Autodesk Inventor part; units mm, degrees
ref_plane "YZ Plane" through (0, 0, 0) normal (1, 0, 0) x (0, 1, 0)
ref_plane "XZ Plane" through (0, 0, 0) normal (0, 1, 0) x (-1, 0, 0)
ref_plane "XY Plane" through (0, 0, 0) normal (0, 0, 1) x (1, 0, 0)
ref_plane "Plano de trabajo1" through (0, 0, 0) normal (0, 0, -1) x (-1, 0, 0)
sketch "Boceto4" plane through (0, 0, 0) normal (0, 0, -1) x (-1, 0, 0)
  circle A0 centre (0, 0) radius 5
  circle A1 centre (0, 0) radius 10
  dimension "d16" = 20
extrude "Extrusión2" add sketch "Boceto4" along normal blind 40
sketch "Boceto5" plane through (0, 0, -40) normal (0, 0, -1) x (-1, 0, 0)
  arc A0 (-15, 0) -> (15, 0) centre (0, 0) ccw
  line L0 (-72.8349, 131.1538) -> (-42.8349, 79.1923)
  line L1 (-47.1651, 76.6923) -> (-77.1651, 128.6538)
  arc A1 (-72.8349, 131.1538) -> (-77.1651, 128.6538) centre (-75, 129.9038) ccw
  arc A2 (-70.4175, 131.9041) -> (-79.3301, 127.4038) centre (-75, 129.9038) ccw
  arc A3 (-47.1651, 76.6923) -> (-42.8349, 79.1923) centre (-45, 77.9423) ccw
  arc A4 (-15, 0) -> (15, 0) centre (0, 0) ccw
  arc A5 (-13.6856, -6.1404) -> (12.4137, 8.4202) centre (0, 0) ccw
  line L2 (-79.3301, 127.4038) -> (-13.2209, -7.0857)
  line L3 (-70.4175, 131.9041) -> (12.5, 8.2916)
  circle A6 centre (0, 0) radius 5
  point P0 (-13.2209, -7.0857)
  point P1 (15, 0)
  point P2 (12.5, 8.2916)
extrude "Extrusión3" add sketch "Boceto5" along normal blind 3 contours L2 A2 L3 A5 A0
sketch "Boceto10" plane through (0, 0, 0) normal (0, 0, -1) x (-1, 0, 0)
  arc A0 (-10, 0) -> (10, 0) centre (0, 0) ccw
  circle A1 centre (0, 0) radius 10
  line L0 (-10, 0) -> (-10, 10)
  line L1 (-10, 10) -> (10, 10)
  line L2 (10, 10) -> (10, 0)
  circle A2 centre (0, 0) radius 5
  dimension "d29" = 10
extrude "Extrusión5" add sketch "Boceto10" against normal blind 10
sketch "Boceto11" plane through (-10, 10, 0) normal (0, 1, 0) x (1, 0, 0)
  circle A0 centre (10, -5) radius 5
  point P0 (10, 0)
extrude "Extrusión6" add sketch "Boceto11" along normal blind 480
sketch "Boceto12" plane through (0, 490, 5) normal (0, 1, 0) x (1, 0, 0)
  arc A0 (25, 0) -> (-25, 0) centre (0, 0) ccw
  line L0 (25, 0) -> (-25, 0)
  point P0 (0, 5)
revolve "Revolución1" add sketch "Boceto12" angle 360 about axis through (25, 490, 5) along (-1, 0, 0)
properties part number "Palanca"
The listing builds one solid part. Answer for the finished solid, in the listing's coordinates (mm). A direction names the side the tool comes from. Coordinates: 2 decimals unless noted, no trailing zeros. Write each loop counter-clockwise with the first axis right and the second up, starting at its lowest first coordinate (ties: lowest second). Pieces come first, ordered by that corner, then holes. Notation, with made-up numbers: (-37, -31.75) - (-13, -31.75) arc R27 cw to (-13, 3.25) - close; hole circle Ø6 at (54.5, 16.5). An arc over 180 degrees is marked (long way). Put each result on its own line as item: value.
1. The part is cut by section D-D on z = -15.5. Give the vertices of the cut face in (x, y), plus the area to 3 significant figures.
Answer sheet:
outline: circle Ø28.62 at (0, 490); circle Ø20 at (0, 0); hole circle Ø10 at (0, 0)
area: 879 mm^2
2. The part is cut by section A-A on z = 5. Give the vertices of the cut face in (x, y), plus the area to 3 significant figures.
Answer sheet:
outline: (-10, 0) arc R10 ccw to (10, 0) - (10, 10) - (5, 10) - (5, 465.51) arc R25 ccw (long way) to (-5, 465.51) - (-5, 10) - (-10, 10) - close; hole circle Ø10 at (0, 0)
area: 6,790 mm^2
3. Determine the mould class of faces 1 (the face through (-8, 8, 0)), 2 (the face through (29.582, 71.027, -41.479)), 3 (the face through (1.08, -4.88, -16.87)) for opening direction X: pulls with the +X half, pulls with the -X half, needs draft (parallel to the pull), parting line crosses it, or undercut.
Answer sheet:
face 1: needs draft
face 2: pulls with the -X half
face 3: undercut
4. The part is cut by section B-B on x = 60. Give the vertices of the cut face in (y, z).
Answer sheet:
outline: (88.08, -43) - (98.92, -43) - (98.92, -40) - (88.08, -40) - close; (108.92, -43) - (116.37, -43) - (116.37, -40) - (108.92, -40) - close
5. Find the intervals of material crossed by line 1 along Y through (x, z) = (0, -6.5); line 2 along Y through (x, z) = (0, -17); line 3 along Y through (x, z) = (0, -32), in increasing order. Write a range as from..to.
Answer sheet:
line 1: y = -10..-5, 5..10, 467.8..512.2
line 2: y = -10..-5, 5..10, 478.13..501.87
line 3: y = -10..-5, 5..10
6. Flat-ended cylindrical pins translate along their axes: pin 1 Ø2 at (x, y) = (-1.5, 318) entering from +Z; pin 2 Ø8 at (x, z) = (-13, 4.5) entering from -Y; pin 3 Ø11 at (x, z) = (-7, 4) entering from +Y; pin 4 Ø6 at (x, z) = (21.5, -35) entering from -Y. Find the tip coordinate at first contact, or state that the pin passes through.
Answer sheet:
pin 1: stops at z = 9.97
pin 2: stops at y = -4.36
pin 3: stops at y = 514.95
pin 4: passes through
7. A tool of negligible diameter and unlimited length cuts with its end or side. For faces 4 (the face through (-2, 5, 10)), 5 (the face through (8, 8, 0)), 6 (the face through (58.045, 105.537, -41.479)), from which of +Z, -Z, +X, -X, +Y, -Y can it reach the whole face along a straight path? Write none if from no direction.
Answer sheet:
face 4: +Z, +X, -X, -Y
face 5: +X
face 6: +Z, -Z
8. The part is cut by section C-C on y = 38. Give the vertices of the cut face in (x, z).
Answer sheet:
outline: circle Ø10 at (0, 5); (7.43, -43) - (35.38, -43) - (35.38, -40) - (7.43, -40) - close
